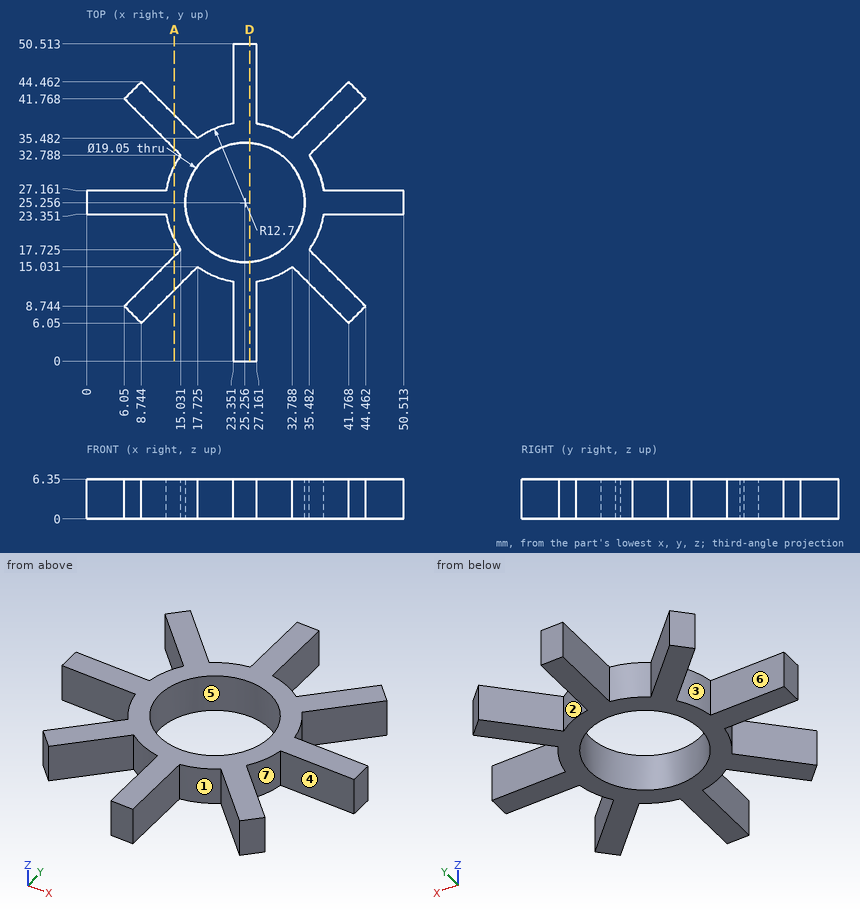
Job drawing, mm, ordinate dimensions from the low corner. One solid piece. A direction names the side the tool comes from. Round coordinates to 2 decimals unless told otherwise and drop trailing zeros. Loops run counter-clockwise (first coordinate to the right, second up) from the corner with the lowest first, then second, coordinate; pieces in that order, holes last.
(1) Cut at D-D (x = 26). Give the cut face in (y, z), plus the area to 3 significant figures.
(2) Which spindle directions (+Z, -Z, +X, -X, +Y, -Y) get a long thin tool onto all of the face, cutting with end or side? Do the marked faces 1, 2, 3 and 4. Say none if no direction does.
(3) Two-plate mould, pull along X, no slides. Class the marked faces 5, 6 and 7: +X half, -X half, draft (parallel to the pull), parting line (faces both ways), or undercut.
(4) Wall check: line 1 along X through (y, z) = (29.5, 4) (1 decimal); line 2 along X through (y, z) = (47.5, 1.25); line 3 along X through (y, z) = (17, 3) (1 decimal). Give the ranges that are in metal, low to high.
(5) Cut at A-A (x = 14). State how many separate pieces and enclosed holes the cut face has, plus the area to 3 significant figures.
(6) Drop flat-ended pins along their axis: pin 1 (1 mm diameter, centred on x = 16, z = 0.5, fed in from +Y) (1 decimal); pin 2 (3 mm diameter, centred on x = 3.5, z = 4, fed in from +Y); pin 3 (3 mm diameter, centred on y = 5.5, z = 3.5, fed in from +X). Give the stop position or say it passes through.
Findings below:
1. outline: (0, 0) - (15.76, 0) - (15.76, 6.35) - (0, 6.35) - close; (34.75, 0) - (50.51, 0) - (50.51, 6.35) - (34.75, 6.35) - close
1. area: 200 mm2
2. face 1: +Z, -Z, -Y
2. face 2: +Z, -Z, +Y
2. face 3: +Z, -Z, -X
2. face 4: +Z, -Z, +X
3. face 5: undercut
3. face 6: draft
3. face 7: +X half
4. line 1: x = 13.3 to 16.7, 33.8 to 37.2
4. line 2: x = 23.35 to 27.16
4. line 3: x = 14.3 to 20.5, 30 to 36.2
5. separate pieces: 3
5. enclosed holes: 0
5. area: 143 mm2
6. pin 1: stops at y = 37.7
6. pin 2: stops at y = 27.16
6. pin 3: stops at x = 42.72
